Check sheet for the modelled part. Datum: model origin and axes. Units: mm. A direction names the side the tool comes from. Round coordinates to 2 decimals unless told otherwise and drop trailing zeros. Write each loop counter-clockwise with the first axis right and the second up, starting at its lowest first coordinate (ties: lowest second). Pieces come first, ordered by that corner, then holes. Notation, with made-up numbers: (-6.75, 66.25) - (8.25, 66.25) arc R10 ccw to (8.25, 75.25) - close; hole circle Ø9 at (3, 71). An arc over 180 degrees is marked (long way). Use one line per item in the form item = value. Start each with the question number.
1) Scan lines: probe 1 along X at (y, z) = (13, -33); probe 2 along Y at (x, z) = (20.5, -8); probe 3 along Y at (x, z) = (41.5, 7). Record each from-to range of solid material in increasing order.
2) Set-up check for faces 4 (the face through (38, 23, 11.346)), 5 (the face through (38, 23, -11.346)), 6 (the face through (38, 43.946, 0)), 7 (the face through (38, 3.445, 0)), 8 (the face through (17.887, 109.236, 9.418)): record each of +Z, -Z, +X, -X, +Y, -Y from which the full face is reachable in a straight line by a thin tool's end or side.
3) Section check A-A (x = 45.5). Record the boundary of the cut face in (y, z).
4) Gauge pin test, flat ends, axial feed: P1, Ø1.5, axis at y = 81.5, z = 30, coming from the +X side; P2, Ø25, axis at x = 44, z = 5.5, coming from the +Y side; P3, Ø6, axis at x = 13, z = 36, coming from the +Y side. Record the tip position at first contact, or that the pin passes through.
5) Draft check along Z on faces 1 (the face through (50.8, 23, 0)), 2 (the face through (12.59, 9.5, -41.36)), 3 (the face through (10.16, 79, 0)). Enter one of: +Z half, -Z half, draft (parallel to the pull), parting line (faces both ways), or undercut.
from build123d import *

# Parameters (mm, degrees)
F1_DEPTH = 25.4
F3_W     = 40.501038
F3_H     = 22.692132
F4_DEPTH = 25.4
F2_R     = 31.353538
F5_DEPTH = 15.24
F6_R     = 21.689952
F7_DEPTH = 25.4
F8_R     = 5.08


with BuildPart() as f1:
    # F0 (on Right) → F1 (new body)
    with BuildSketch(Plane.YZ):
        with BuildLine():
            ThreePointArc((133.647867, 0), (113.743156, 42.025772), (68.617132, 53.250967))
            ThreePointArc((68.617132, 53.250967), (25.012127, 0), (68.617132, -53.250967))
            ThreePointArc((68.617132, -53.250967), (113.743156, -42.025772), (133.647867, 0))
        make_face()
        with BuildLine():
            ThreePointArc((-47.991263, -29.79205), (-22.744834, -23.511947), (-11.608846, 0))
            ThreePointArc((-11.608846, 0), (-22.744834, 23.511947), (-47.991263, 29.79205))
            ThreePointArc((-47.991263, 29.79205), (-72.386735, 0), (-47.991263, -29.79205))
        make_face()
        with BuildLine():
            ThreePointArc((-47.991263, 29.79205), (-22.744834, 23.511947), (-11.608846, 0))
            ThreePointArc((-11.608846, 0), (-22.744834, -23.511947), (-47.991263, -29.79205))
            Line((-47.991263, -29.79205), (68.617132, -53.250967))
            ThreePointArc((68.617132, -53.250967), (25.012127, 0), (68.617132, 53.250967))
            Line((68.617132, 53.250967), (-47.991263, 29.79205))
        make_face()
    extrude(amount=F1_DEPTH)

    # F3 (on face) → F4 (join)
    with BuildSketch(Plane.YZ.offset(25.4)):
        with Locations((23.695795, 0)):
            Rectangle(F3_W, F3_H)
    extrude(amount=F4_DEPTH)

    # F2 (on face) → F5 (cut)
    with BuildSketch(Plane.YZ.offset(25.4)):
        with Locations((79.329997, 0)):
            Circle(F2_R)
    extrude(amount=-F5_DEPTH, mode=Mode.SUBTRACT)

    # F6 (on face) → F7 (cut)
    with BuildSketch(Plane.YZ.offset(25.4)):
        with Locations((-41.99779, 0)):
            Circle(F6_R)
    extrude(amount=-F7_DEPTH, mode=Mode.SUBTRACT)

    # F8
    f8_edges = [f1.edges().sort_by_distance(p)[0] for p in [
        (0, -72.386735, 0),
        (12.7, -47.991263, -29.79205),
        (25.4, -72.386735, 0),
        (12.7, -47.991263, 29.79205),
    ]]
    fillet(f8_edges, radius=F8_R)


solid = f1.part
Results are:
q1.probe_1 = 0 to 25.4
q1.probe_2 = -71.31 to -62.16, -21.84 to 49.01, 109.65 to 133.05
q1.probe_3 = 3.45 to 43.95
q2.face_4 = +Z, +X, +Y, -Y
q2.face_5 = -Z, +X, +Y, -Y
q2.face_6 = +Z, -Z, +X, +Y
q2.face_7 = +Z, -Z, +X, -Y
q2.face_8 = +X
q3.outline = (3.45, -11.35) - (43.95, -11.35) - (43.95, 11.35) - (3.45, 11.35) - close
q4.P1 = 10.16
q4.P2 = 43.95
q4.P3 = 122.47
q5.face_1 = draft
q5.face_2 = -Z half
q5.face_3 = undercut
